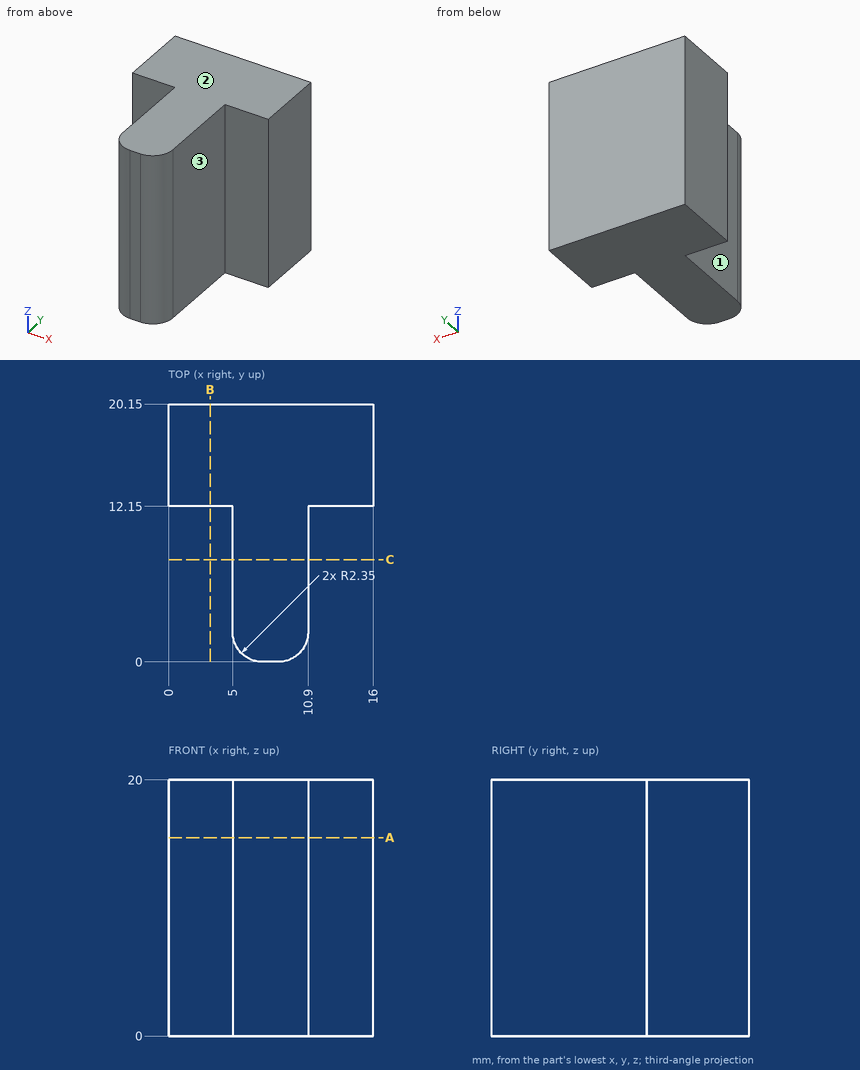
Here's the drawing with two shaded views (mm, measured from the low corner). I have some questions. A direction names the side the tool comes from. Coordinates: 2 decimals unless noted, no trailing zeros. Loops run counter-clockwise (first coordinate to the right, second up) from the corner with the lowest first, then second, coordinate; pieces in that order, holes last. Notation, with made-up numbers: (77, 86.25) -> (93, 86.25) arc R15 cw to (93, 98.25) -> close; hole circle Ø9 at (35, -13). An arc over 180 degrees is marked (long way). Answer in a Markdown table with one row per item.
(1) For the marked faces 1, 2 and 3, which set-ups out of +Z, -Z, +X, -X, +Y, -Y let a thin tool reach every point of the face, with its end or its side?
Results found:
| item | result |
|---|---|
| face 1 | +Z, -Z, -X, -Y |
| face 2 | +Z, +X, -X, +Y, -Y |
| face 3 | +Z, -Z, +X, -Y |
(2) Will these pins go through, and if not, where does the flat tip stop? pin 1 Ø5 at (y, z) = (7.5, 9.5) entering from +X; pin 2 Ø2.5 at (x, z) = (13, 8) entering from -Y; pin 3 Ø3 at (x, z) = (5.5, 3.5) entering from -Y.
Results found:
| item | result |
|---|---|
| pin 1 | stops at x = 10.9 |
| pin 2 | stops at y = 12.15 |
| pin 3 | stops at y = 0.03 |
(3) Imagine slicing it at B-B (x = 3.25). List the corners of the cut face in (y, z) for me.
Results found:
| item | result |
|---|---|
| outline | (12.15, 0) -> (20.15, 0) -> (20.15, 20) -> (12.15, 20) -> close |
(4) Imagine slicing it at A-A (z = 15.5). List the corners of the cut face in (x, y) for me, plus the area to 3 significant figures.
Results found:
| item | result |
|---|---|
| outline | (0, 12.15) -> (5, 12.15) -> (5, 2.35) arc R2.35 ccw to (7.35, 0) -> (8.55, 0) arc R2.35 ccw to (10.9, 2.35) -> (10.9, 12.15) -> (16, 12.15) -> (16, 20.15) -> (0, 20.15) -> close |
| area | 197 mm^2 |
(5) If I drill on probe 1 along Y at (x, z) = (0.75, 3); probe 2 along X at (y, z) = (8, 13.5); probe 3 along Y at (x, z) = (7.25, 9.5), over which ranges is the centre line in solid material (lowest first)?
Results found:
| item | result |
|---|---|
| probe 1 | y = 12.15 to 20.15 |
| probe 2 | x = 5 to 10.9 |
| probe 3 | y = 0 to 20.15 |
(6) Imagine slicing it at C-C (y = 8). List the corners of the cut face in (x, z) for me.
Results found:
| item | result |
|---|---|
| outline | (5, 0) -> (10.9, 0) -> (10.9, 20) -> (5, 20) -> close |
